```python
from build123d import *

# Parameters (mm, degrees)
SKETCH1_W           = 550
SKETCH1_H           = 25.4
BOSS_EXTRUDE1_DEPTH = 25.4
SKETCH2_W           = 23
SKETCH2_H           = 23
CUT_EXTRUDE1_DEPTH  = 550
CUT_EXTRUDE2_DEPTH  = 25.4


with BuildPart() as part:
    # Sketch1 → Boss-Extrude1 (new body)
    with BuildSketch(Plane(origin=(0, 0, 0), x_dir=(1, 0, 0), z_dir=(0, 1, 0))):
        with Locations((275, 12.7)):
            Rectangle(SKETCH1_W, SKETCH1_H)
    extrude(amount=BOSS_EXTRUDE1_DEPTH)

    # Sketch2 → Cut-Extrude1 (cut)
    with BuildSketch(Plane(origin=(550, 0, 0), x_dir=(0, 0, -1), z_dir=(1, 0, 0))):
        with Locations((12.7, 12.7)):
            Rectangle(SKETCH2_W, SKETCH2_H)
    extrude(amount=-CUT_EXTRUDE1_DEPTH, mode=Mode.SUBTRACT)

    # Sketch3 → Cut-Extrude2 (cut)
    with BuildSketch(Plane(origin=(0, 25.4, 0), x_dir=(1, 0, 0), z_dir=(0, 1, 0))):
        Polygon((0, 0), (25.4, 25.4), (0, 25.4), align=None)
        Polygon((550, 0), (524.6, 25.4), (550, 25.4), align=None)
    extrude(amount=-CUT_EXTRUDE2_DEPTH, mode=Mode.SUBTRACT)


solid = part.part
```
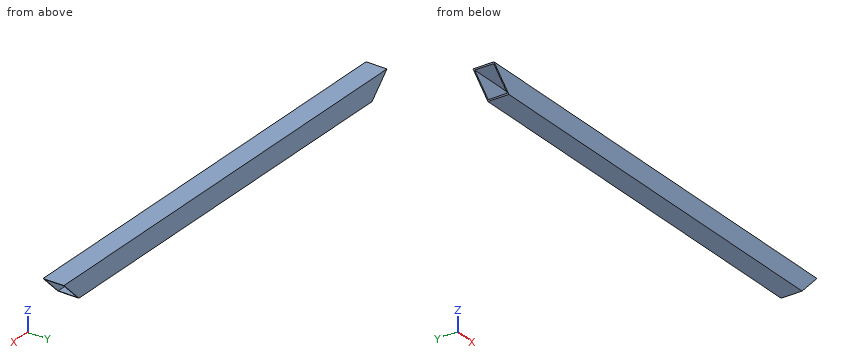
Can you work these out from the model? Positions are in its coordinate system, mm. Coordinates: 2 decimals unless noted, no trailing zeros. Loops run counter-clockwise (first coordinate to the right, second up) from the corner with the lowest first, then second, coordinate; pieces in that order, holes last. Notation, with made-up numbers: M -32,-18.75 L -10,-18.75 A17 ccw -10,13.25 Z; hole C 56,68 d3. An arc over 180 degrees is marked long. Put each result on its own line as item: value. Start each with the question number.
(1) Imagine slicing it at B-B on x = 79.5. List the corners of the cut face in (y, z) for me, and give its area (3 significant figures).
(2) I need wall thicknesses on probe 1 along Y at (x, z) = (37.5, -20.5); probe 2 along Z at (x, y) = (273, 2.75); probe 3 along X at (y, z) = (11.75, -24.5). Which ranges of each line are inside material? Lowest first, please.
(3) Imagine slicing it at C-C on z = -6.5. List the corners of the cut face in (x, y) for me.
(4) Will this pin go through, and if not, where does the flat tip stop? pin 1 Ø7 at (x, y) = (279.5, 9) entering from +Z.
(5) Imagine slicing it at A-A on y = 17.5. List the corners of the cut face in (x, z) for me, and give its area (3 significant figures).
Worked answers:
1. outline: M 0,-25.4 L 25.4,-25.4 L 25.4,0 L 0,0 Z; hole M 1.2,-24.2 L 24.2,-24.2 L 24.2,-1.2 L 1.2,-1.2 Z
1. area: 116 mm2
2. probe 1: y = 0 to 1.2, 24.2 to 25.4
2. probe 2: z = -25.4 to -24.2, -1.2 to 0
2. probe 3: x = 24.5 to 525.5
3. outline: M 6.5,0 L 543.5,0 L 543.5,1.2 L 6.5,1.2 Z; M 6.5,24.2 L 543.5,24.2 L 543.5,25.4 L 6.5,25.4 Z
4. pin 1: stops at z = 0
5. outline: M 0,0 L 1.2,-1.2 L 548.8,-1.2 L 550,0 Z; M 24.2,-24.2 L 25.4,-25.4 L 524.6,-25.4 L 525.8,-24.2 Z
5. area: 1,260 mm2
